Here's how the part is built. I have some questions about the finished solid (model axes, mm). Face numbers are marked on the shaded views. A direction names the side the tool comes from. Coordinates: 2 decimals unless noted, no trailing zeros. Loops run counter-clockwise (first coordinate to the right, second up) from the corner with the lowest first, then second, coordinate; pieces in that order, holes last. Notation, with made-up numbers: (-39.5, 56.5) - (1.5, 56.5) arc R8 ccw to (1.5, 65.5) - close; hole circle Ø1 at (-34.5, 38.25). An arc over 180 degrees is marked (long way). Use a Markdown table: item, result.
```python
from build123d import *

# Parameters (mm, degrees)
BOSS_EXTRUDE1_DEPTH  = 19.812
SKETCH2_R            = 2.249999945
CUT_EXTRUDE1_DEPTH   = 46.597067399
BOSS_EXTRUDE2_DEPTH  = 2.699999934
SKETCH12_R           = 6.549999981
BOSS_EXTRUDE8_DEPTH  = 1.159999966
SKETCH13_R           = 5.334999998
BOSS_EXTRUDE9_DEPTH  = 0.65999995
SKETCH14_R           = 2.975000019
BOSS_EXTRUDE11_DEPTH = 4.000000128


with BuildPart() as part:
    # Sketch1 → Boss-Extrude1 (new body)
    with BuildSketch(Plane(origin=(0, 0, 0), x_dir=(1, 0, 0), z_dir=(0, 1, 0))):
        Polygon((-20.399999967, -18.174999972), (20.399999967, -18.174999972), (20.399999967, 10.124999816), (27.164999899, 10.124999816), (27.164999899, 12.624999896), (20.399999967, 12.624999896), (20.399999967, 18.174999972), (-20.399999967, 18.174999972), (-20.399999967, 12.624999896), (-27.164999899, 12.624999896), (-27.164999899, 10.124999816), (-20.399999967, 10.124999816), align=None)
    extrude(amount=BOSS_EXTRUDE1_DEPTH)

    # Sketch2 → Cut-Extrude1 (cut, through all)
    with BuildSketch(Plane(origin=(0, 0, -12.624999896), x_dir=(-1, 0, 0), z_dir=(0, 0, -1))):
        with Locations((25.009999891, 4.869999912)):
            Circle(SKETCH2_R)
        with Locations((25.009999891, 14.942000088)):
            Circle(SKETCH2_R)
        with Locations((-25.009999891, 4.869999912)):
            Circle(SKETCH2_R)
        with Locations((-25.009999891, 14.942000088)):
            Circle(SKETCH2_R)
    extrude(amount=-CUT_EXTRUDE1_DEPTH, mode=Mode.SUBTRACT)

    # Sketch3 → Boss-Extrude2 (add)
    with BuildSketch(Plane(origin=(0, 0, -18.174999972), x_dir=(-1, 0, 0), z_dir=(0, 0, -1))):
        with BuildLine():
            Line((-14.650000037, 18.80599998), (-14.650000037, 1.00600002))
            Line((-14.650000037, 1.00600002), (6.098630297, 1.00600002))
            ThreePointArc((6.098630297, 1.00600002), (0.559999979, 9.906), (6.098630297, 18.80599998))
            Line((6.098630297, 18.80599998), (-14.650000037, 18.80599998))
        make_face()
        with BuildLine():
            ThreePointArc((6.098630297, 18.80599998), (0.559999979, 9.906), (6.098630297, 1.00600002))
            ThreePointArc((6.098630297, 1.00600002), (7.974875683, 0.307523445), (9.953156655, 0))
            Line((9.953156655, 0), (11.006843291, 0))
            ThreePointArc((11.006843291, 0), (17.678356924, 3.08030904), (20.399999967, 9.906))
            ThreePointArc((20.399999967, 9.906), (17.678356924, 16.73169096), (11.006843291, 19.812))
            Line((11.006843291, 19.812), (9.953156655, 19.812))
            ThreePointArc((9.953156655, 19.812), (7.974875683, 19.504476555), (6.098630297, 18.80599998))
        make_face()
    extrude(amount=BOSS_EXTRUDE2_DEPTH)

    # Sketch12 → Boss-Extrude8 (add)
    with BuildSketch(Plane(origin=(0, 0, -20.874999906), x_dir=(-1, 0, 0), z_dir=(0, 0, -1))):
        with Locations((10.479999973, 9.906)):
            Circle(SKETCH12_R)
    extrude(amount=BOSS_EXTRUDE8_DEPTH)

    # Sketch13 → Boss-Extrude9 (add)
    with BuildSketch(Plane(origin=(0, 0, -22.034999872), x_dir=(-1, 0, 0), z_dir=(0, 0, -1))):
        with Locations(Location((10.479999973, 9.906, 0), (0, 0, 180))):
            Circle(SKETCH13_R)
    extrude(amount=BOSS_EXTRUDE9_DEPTH)

    # Sketch14 → Boss-Extrude11 (add)
    with BuildSketch(Plane(origin=(0, 0, -22.694999822), x_dir=(-1, 0, 0), z_dir=(0, 0, -1))):
        with Locations((10.479999973, 9.906)):
            Circle(SKETCH14_R)
    extrude(amount=BOSS_EXTRUDE11_DEPTH)


solid = part.part
```
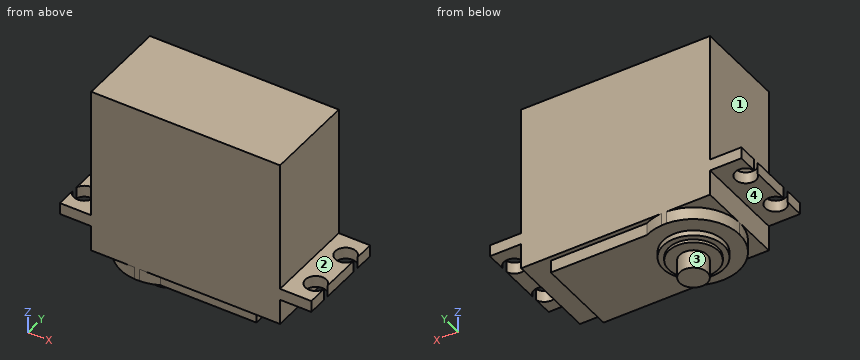
Q1. I want a section at A-A, the plane z = -12. Write out the boundary of the cut face in (x, y) (3 decimals), then the cut area to 3 significant figures.
Check values:
| item | result |
|---|---|
| outline | (-27.165, 0) - (27.165, 0) - (27.165, 4.223) arc R2.25 cw (long way) to (27.165, 5.517) - (27.165, 14.295) arc R2.25 cw (long way) to (27.165, 15.589) - (27.165, 19.812) - (-27.165, 19.812) - (-27.165, 15.589) arc R2.25 cw (long way) to (-27.165, 14.295) - (-27.165, 5.517) arc R2.25 cw (long way) to (-27.165, 4.223) - close |
| area | 1,010 mm^2 |
Q2. I want a section at C-C, the plane x = 5.5. Write out the boundary of the cut face in (y, z) (3 decimals), then the cut area to 3 significant figures.
Check values:
| item | result |
|---|---|
| outline | (0, -18.175) - (1.006, -18.175) - (1.006, -20.875) - (18.806, -20.875) - (18.806, -18.175) - (19.812, -18.175) - (19.812, 18.175) - (0, 18.175) - close |
| area | 768 mm^2 |
Q3. I want a section at D-D, the plane y = 7.75. Write out the boundary of the cut face in (x, z) (3 decimals).
Check values:
| item | result |
|---|---|
| outline | (-27.165, -12.625) - (-20.4, -12.625) - (-20.4, -18.175) - (-20.163, -18.175) - (-20.163, -20.875) - (-16.665, -20.875) - (-16.665, -22.035) - (-15.36, -22.035) - (-15.36, -22.695) - (-12.53, -22.695) - (-12.53, -26.695) - (-8.43, -26.695) - (-8.43, -22.695) - (-5.6, -22.695) - (-5.6, -22.035) - (-4.295, -22.035) - (-4.295, -20.875) - (14.65, -20.875) - (14.65, -18.175) - (20.4, -18.175) - (20.4, -12.625) - (27.165, -12.625) - (27.165, -10.125) - (20.4, -10.125) - (20.4, 18.175) - (-20.4, 18.175) - (-20.4, -10.125) - (-27.165, -10.125) - close |
Q4. Will these pins go through, and if not, where does the flat tip stop? P1, Ø5, axis at x = -25.01, y = 4.87, coming from the -Z side (3 decimals); P2, Ø1, axis at y = 12.5, z = 11.5, coming from the -X side; P3, Ø1.7, axis at y = 14.5, z = -14.5, coming from the +X side; P4, Ø4, axis at x = -25.01, y = 14.942, coming from the +Z side.
Check values:
| item | result |
|---|---|
| P1 | z = -12.625 |
| P2 | x = -20.4 |
| P3 | x = 20.4 |
| P4 | through |
Q5. I want a section at B-B, the plane x = 25.01. Write out the boundary of the cut face in (y, z) (3 decimals).
Check values:
| item | result |
|---|---|
| outline | (0, -12.625) - (2.62, -12.625) - (2.62, -10.125) - (0, -10.125) - close; (7.12, -12.625) - (12.692, -12.625) - (12.692, -10.125) - (7.12, -10.125) - close; (17.192, -12.625) - (19.812, -12.625) - (19.812, -10.125) - (17.192, -10.125) - close |
Q6. Which directions (+Z, -Z, +X, -X, +Y, -Y) give clear straight access to the entire face, cutting with the end or side of a thin tool? Please do the marked faces 1, 2, 3 and 4.
Check values:
| item | result |
|---|---|
| face 1 | +Z, -X, +Y, -Y |
| face 2 | +Z, +X, +Y, -Y |
| face 3 | -Z |
| face 4 | -Z, -X, +Y, -Y |
Q7. Please list where these lines run through material, in increasing order: L1, parallel to Y at x = -25.01, z = -11.95; L2, parallel to Z at x = 22, y = 1 (3 decimals); L3, parallel to Z at x = -14.5, y = 17.5 (3 decimals). Write a range as from..to.
Check values:
| item | result |
|---|---|
| L1 | 0..2.62, 7.12..12.69, 17.19..19.81 |
| L2 | -12.625..-10.125 |
| L3 | -20.875..18.175 |
